Geometry check sheet. Reference: the model listing, model coordinates, mm. Face numbers are marked on the shaded views. A direction names the side the tool comes from. Coordinates: 2 decimals unless noted, no trailing zeros. Write each loop counter-clockwise with the first axis right and the second up, starting at its lowest first coordinate (ties: lowest second). Pieces come first, ordered by that corner, then holes.
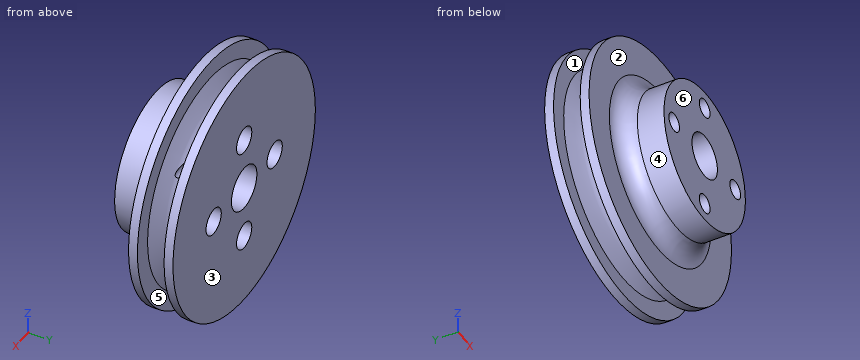
from build123d import *

# Parameters (mm, degrees)
SKETCH_1_R               = 8
EXTRUDE_1_DEPTH          = 5
SKETCH_4_R               = 1.5
CUT_EXTRUDE_1_DEPTH      = 5
SKETCH_5_R               = 1.05
CUT_EXTRUDE_2_DEPTH      = 5
CUT_EXTRUDE_3_DEPTH      = 20.697715725
CUT_EXTRUDE_3_DEPTH_BACK = 20.697715725
SKETCH_6_R               = 0.75
FILLET_1_R               = 2
SKETCH_7_R               = 2.5
CUT_EXTRUDE_4_DEPTH      = 18.691806177
SKETCH_8_W               = 2
SKETCH_8_H               = 1


with BuildPart() as part:
    # 草图1 → 凸台-拉伸1 (new body)
    with BuildSketch(Plane(origin=(0, 0, 0), x_dir=(1, 0, 0), z_dir=(0, 1, 0))):
        with Locations(Location((0, 0, 0), (0, 0, 270))):
            Circle(SKETCH_1_R)
    extrude(amount=EXTRUDE_1_DEPTH)

    # 草图3 → 旋转3 (revolve)
    with BuildSketch(Plane.XY, mode=Mode.PRIVATE) as revolve_3_sk:
        with BuildLine():
            Line((2.5, 5), (12, 5))
            Line((12, 5), (12, 6))
            add(Edge.make_bspline(
                [(12, 6), (11.881605513, 6.037686136), (11.643847391, 6.113366384), (11.1308123, 6.277999279), (10.853848161, 6.374268454), (10.462432208, 6.511227783), (10.343110433, 6.559604769), (10.19237694, 6.616697566), (10.135568567, 6.640570799), (10.044493212, 6.677585871), (9.943739799, 6.720706003), (9.809699725, 6.780371733), (9.648775717, 6.858112274), (9.471041518, 6.953541858), (9.30348757, 7.060847742), (9.170715349, 7.168533862), (9.081288373, 7.270836083), (9.034264055, 7.349098369), (9.00966007, 7.414359694), (8.999065655, 7.473026617), (8.999342857, 7.529783688), (9.010470802, 7.588482504), (9.035781555, 7.653997439), (9.08372319, 7.732478484), (9.154743932, 7.812639974), (9.243856794, 7.890764576), (9.36325959, 7.977520225), (9.480401778, 8.049948999), (9.59976532, 8.115407144), (9.725024816, 8.178944598), (9.843468468, 8.234393018), (9.962029893, 8.288066069), (10.093902347, 8.342284824), (10.180119226, 8.378587138), (10.347165548, 8.442047118), (10.468262515, 8.490865615), (10.857491167, 8.626989754), (11.133661478, 8.72292094), (11.645360185, 8.887115159), (11.882008148, 8.962442027), (12, 9)],
                knots=[0.083325581, 0.083325581, 0.083325581, 0.083325581, 0.083325581, 0.155200362, 0.227075164, 0.263012583, 0.298950001, 0.307934351, 0.316918701, 0.32590305, 0.3348874, 0.352856099, 0.370824799, 0.396081378, 0.421337957, 0.449866264, 0.4667317, 0.47810977, 0.48654791, 0.493647494, 0.50018096, 0.506692176, 0.513761649, 0.522297603, 0.533856047, 0.55081559, 0.565113209, 0.579410828, 0.604781909, 0.61746745, 0.63015299, 0.648060561, 0.665968131, 0.683875702, 0.692829487, 0.701783273, 0.737598478, 0.773413683, 0.845044069, 0.916674419, 0.916674419, 0.916674419, 0.916674419, 0.916674419], degree=4))
            Line((12, 9), (12, 10))
            Line((12, 10), (2.5, 10))
            Line((2.5, 10), (2.5, 5))
        make_face()
    revolve(revolve_3_sk.sketch.rotate(Axis((0, 11, 0), (0, -1, 0)), 90), axis=Axis((0, 11, 0), (0, -1, 0)))

    # 草图4 → 切除-拉伸1 (cut)
    with BuildSketch(Plane(origin=(0, 10, 0), x_dir=(1, 0, 0), z_dir=(0, 1, 0))):
        with Locations(Location((0, 6, 0), (0, 0, 180))):
            Circle(SKETCH_4_R)
        with Locations(Location((6, 0, 0), (0, 0, 180))):
            Circle(SKETCH_4_R)
        with Locations(Location((0, -6, 0), (0, 0, 180))):
            Circle(SKETCH_4_R)
        with Locations(Location((-6, 0, 0), (0, 0, 180))):
            Circle(SKETCH_4_R)
    extrude(amount=-CUT_EXTRUDE_1_DEPTH, mode=Mode.SUBTRACT)

    # 草图5 → 切除-拉伸2 (cut)
    with BuildSketch(Plane(origin=(0, 5, 0), x_dir=(1, 0, 0), z_dir=(0, 1, 0))):
        with Locations(Location((0, 6, 0), (0, 0, 180))):
            Circle(SKETCH_5_R)
        with Locations(Location((-6, 0, 0), (0, 0, 180))):
            Circle(SKETCH_5_R)
        with Locations(Location((6, 0, 0), (0, 0, 180))):
            Circle(SKETCH_5_R)
        with Locations(Location((0, -6, 0), (0, 0, 180))):
            Circle(SKETCH_5_R)
    extrude(amount=-CUT_EXTRUDE_2_DEPTH, mode=Mode.SUBTRACT)

    # 草图6 → 切除-拉伸3 (cut, two sides: drawn at the far end of the back side and taken through both)
    with BuildSketch(Plane(origin=(0, 0, 0), x_dir=(0, 0, -1), z_dir=(1, 0, 0)).offset(-CUT_EXTRUDE_3_DEPTH_BACK)):
        with Locations((-6, 7.5)):
            Circle(SKETCH_6_R)
    extrude(amount=CUT_EXTRUDE_3_DEPTH + CUT_EXTRUDE_3_DEPTH_BACK, mode=Mode.SUBTRACT)

    # 圆角1
    fillet_1_edges = [part.edges().sort_by_distance(p)[0] for p in [
        (0, 5, -8),
    ]]
    fillet(fillet_1_edges, radius=FILLET_1_R)

    # 草图7 → 切除-拉伸4 (cut, through all)
    with BuildSketch(Plane(origin=(0, 5, 0), x_dir=(1, 0, 0), z_dir=(0, 1, 0))):
        with Locations(Location((0, 0, 0), (0, 0, 270))):
            Circle(SKETCH_7_R)
    extrude(amount=-CUT_EXTRUDE_4_DEPTH, mode=Mode.SUBTRACT)

    # 草图8 → 旋转4 (revolve)
    with BuildSketch(Plane.XY, mode=Mode.PRIVATE) as revolve_4_sk:
        with Locations((13, 9.5)):
            Rectangle(SKETCH_8_W, SKETCH_8_H)
        with Locations((13, 5.5)):
            Rectangle(SKETCH_8_W, SKETCH_8_H)
    revolve(revolve_4_sk.sketch.rotate(Axis((0, 9, 0), (0, -1, 0)), 180), axis=Axis((0, 9, 0), (0, -1, 0)))


solid = part.part
1. Draft check along Y on the marked faces 4, 5 and 6. Enter one of: released by +Y, released by -Y, zero draft, split by the parting line, or undercut.
Computed values:
face 4: zero draft
face 5: undercut
face 6: released by -Y
2. Sectioned sample at A-A, the plane y = 1.5. Record the boundary of the cut face in (x, z).
Computed values:
outline: circle Ø16 at (0, 0); hole circle Ø2.1 at (-6, 0); hole circle Ø5 at (0, 0); hole circle Ø2.1 at (0, -6); hole circle Ø2.1 at (0, 6); hole circle Ø2.1 at (6, 0)
3. Access from +Z, -Z, +X, -X, +Y, -Y to the whole of each face (thin tool, end or side, straight path). Record for the marked faces 1, 2 and 3.
Computed values:
face 1: none
face 2: -Y
face 3: +Z, -Z, +X, -X, +Y
4. Sectioned sample at B-B, the plane z = 0. Give the number of separate pieces and of enclosed holes in the cut face, and give its area (3 significant figures).
Computed values:
separate pieces: 4
enclosed holes: 0
area: 97.3 mm2
5. Gauge pin test, flat ends, axial feed: pin 1 Ø2.5 at (x, z) = (0, 6) entering from +Y; pin 2 Ø0.9 at (y, z) = (7.5, 6) entering from -X; pin 3 Ø3 at (y, z) = (1.5, -2.5) entering from -X; pin 4 Ø4 at (x, y) = (-6.5, 6) entering from -Z. Record the tip position at first contact, or that the pin passes through.
Computed values:
pin 1: stops at y = 5
pin 2: passes through
pin 3: stops at x = -7.94
pin 4: stops at z = -13.26
6. Sectioned sample at D-D, the plane y = 3.75. Record the boundary of the cut face in (x, z), and give its area (3 significant figures).
Computed values:
outline: circle Ø16.29 at (0, 0); hole circle Ø2.1 at (-6, 0); hole circle Ø5 at (0, 0); hole circle Ø2.1 at (0, -6); hole circle Ø2.1 at (0, 6); hole circle Ø2.1 at (6, 0)
area: 175 mm2
7. Thickness scan on line 1 along Y through (x, z) = (4, 12); line 2 along Z through (x, y) = (-4.75, 7.5); line 3 along Z through (x, y) = (-5.5, 7.25). Record the ranges inside material, lowest first.
Computed values:
line 1: y = 5 to 6, 9 to 10
line 2: z = -7.64 to -0.83, 0.83 to 5.25, 6.75 to 7.64
line 3: z = -7.25 to -1.41, 1.41 to 5.29, 6.71 to 7.25
